The model under review builds one solid part; all positions refer to its coordinate system, in mm. A direction names the side the tool comes from. Round coordinates to 2 decimals unless told otherwise and drop trailing zeros. Write each loop counter-clockwise with the first axis right and the second up, starting at its lowest first coordinate (ties: lowest second). Pieces come first, ordered by that corner, then holes. Notation, with made-up numbers: (-23.5, 8.25) - (24.5, 8.25) arc R14 cw to (24.5, 35.25) - close; hole circle Ø11 at (85, 87.25). An arc over 180 degrees is marked (long way). Write each question's results on one line, items separated by ' | '.
```python
from build123d import *

# Parameters (mm, degrees)
F0_W          = 75
F0_H          = 35
F1_DEPTH      = 3
F4_W          = 10.7173770666
F4_H          = 34.9826700985
F5_DEPTH      = 25
F7_W          = 6
F7_H          = 35
F7_W_2        = 2
F7_H_2        = 28
F8_DEPTH      = 10
F9_DEPTH      = 10
F9_FACE_W     = 6
F9_FACE_H     = 35
F11_W         = 2
F11_H         = 28
F14_DEPTH     = 6
F16_DEPTH     = 25
F17_R         = 2
F18_R         = 0.5
F20_T1_DEPTH  = 12
F20_T4_ANGLE  = 90
F20_T6_ANGLE  = 90
F20_T8_ANGLE  = 90
F20_T10_ANGLE = 90
F21_R         = 1


# Not quite as in the source:
# - a fillet or chamfer that OpenCascade refuses, or shapes differently, is made with other operations: its cross-section is extruded or revolved along the edge and cut away or added
# - a feature of the source that left no trace in its solid (it failed there, or was rolled back) is left out
# - a feature names something its author has since deleted; it is built from what else it names


with BuildPart() as f1:
    # F0 (on Right) → F1 (new body, symmetric)
    with BuildSketch(Plane.YZ):
        with Locations((37.5, 0)):
            Rectangle(F0_W, F0_H)
    extrude(amount=F1_DEPTH, both=True)

    # F4 (on offset) → F5 (cut)
    with BuildSketch(Plane.XZ.offset(-10)):
        Rectangle(F4_W, F4_H)
    extrude(amount=F5_DEPTH, mode=Mode.SUBTRACT)

    # F7 (on face) → F8 (cut)
    with BuildSketch(Plane(origin=(0, 75, 0), x_dir=(-1, 0, 0), z_dir=(0, 1, 0))):
        Rectangle(F7_W, F7_H)
        Rectangle(F7_W_2, F7_H_2, mode=Mode.SUBTRACT)
    extrude(amount=F8_DEPTH, mode=Mode.SUBTRACT)

    # F9 (cut): a face of the model
    f9_faces = [f1.faces().sort_by_distance(p)[0] for p in [
        (0, 75, 0),
    ]]
    extrude(f9_faces, amount=-F9_DEPTH, mode=Mode.SUBTRACT)

    # F9_face (on face) → F12 section 0
    with BuildSketch(Plane(origin=(0, 65, 0), x_dir=(-1, 0, 0), z_dir=(0, 1, 0))):
        Rectangle(F9_FACE_W, F9_FACE_H)
    # F11 (on offset) → F12 section 1
    with BuildSketch(Plane(origin=(0, 75, 0), x_dir=(-1, 0, 0), z_dir=(0, 1, 0))):
        Rectangle(F11_W, F11_H)
    loft()

    # F13 (on Right) → F14 (join, symmetric)
    with BuildSketch(Plane.YZ):
        Polygon((25, 21.5), (0, 21.5), (-25, 21.5), (-25, 0), (-25, -21.5), (0, -21.5), (25, -21.5), (25, 0), align=None)
    extrude(amount=F14_DEPTH, both=True)

    # F15 (on face) → F16 (cut)
    with BuildSketch(Plane(origin=(-6, 0, 0), x_dir=(0, -1, 0), z_dir=(-1, 0, 0))):
        with BuildLine():
            Line((-5, -12.5), (5, -12.5))
            ThreePointArc((5, -12.5), (6.4142135624, -11.9142135624), (7, -10.5))
            Line((7, -10.5), (7, -9.5))
            ThreePointArc((7, -9.5), (6.4142135624, -8.0857864376), (5, -7.5))
            Line((5, -7.5), (-5, -7.5))
            ThreePointArc((-5, -7.5), (-6.4142135624, -8.0857864376), (-7, -9.5))
            Line((-7, -9.5), (-7, -10.5))
            ThreePointArc((-7, -10.5), (-6.4142135624, -11.9142135624), (-5, -12.5))
        make_face()
    extrude(amount=-F16_DEPTH, mode=Mode.SUBTRACT)

    # F17
    f17_edges = [f1.edges().sort_by_distance(p)[0] for p in [
        (6, 0, -7.5),
        (6, -6.414214, -8.085786),
        (6, -7, -10),
        (6, -6.414214, -11.914214),
        (6, 0, -12.5),
        (6, 6.414214, -8.085786),
        (6, 7, -10),
        (6, 6.414214, -11.914214),
        (-6, 0, -7.5),
        (-6, -6.414214, -8.085786),
        (-6, -7, -10),
        (-6, -6.414214, -11.914214),
        (-6, 0, -12.5),
        (-6, 6.414214, -11.914214),
        (-6, 7, -10),
        (-6, 6.414214, -8.085786),
    ]]
    fillet(f17_edges, radius=F17_R)

    # F18
    f18_edges = [f1.edges().sort_by_distance(p)[0] for p in [
        (-6, 0, 21.5),
        (0, -25, 21.5),
        (6, 0, 21.5),
        (0, 25, 21.5),
        (6, 0, -5.5),
        (6, 7.828427, -6.671573),
        (6, -7.828427, -6.671573),
        (6, 9, -10),
        (6, -9, -10),
        (6, 7.828427, -13.328427),
        (6, -7.828427, -13.328427),
        (6, 0, -14.5),
        (6, -25, 0),
        (6, 25, 0),
        (6, 0, -21.5),
        (-6, 0, -5.5),
        (-6, -7.828427, -6.671573),
        (-6, 7.828427, -6.671573),
        (-6, -9, -10),
        (-6, 9, -10),
        (-6, -7.828427, -13.328427),
        (-6, 7.828427, -13.328427),
        (-6, 0, -14.5),
        (-6, 25, 0),
        (-6, -25, 0),
        (-6, 0, -21.5),
    ]]
    fillet(f18_edges, radius=F18_R)

    # F19: F1 across plane


with BuildPart() as f1_1:
    add(f1.part)
    add(f1.part.mirror(Plane.XZ))

    # F20: fillet of radius 1 on 2 edges, made by hand

    # F20_s2 → F20_t1 (cut)
    with BuildSketch(Plane.YZ.offset(-6)):
        with BuildLine():
            ThreePointArc((25, -20.5), (24.7071067812, -21.2071067812), (24, -21.5))
            Line((24, -21.5), (25, -21.5))
            Line((25, -21.5), (25, -20.5))
        make_face()
        with BuildLine():
            ThreePointArc((-25, -20.5), (-24.7071067812, -21.2071067812), (-24, -21.5))
            Line((-24, -21.5), (-25, -21.5))
            Line((-25, -21.5), (-25, -20.5))
        make_face()
    extrude(amount=F20_T1_DEPTH, mode=Mode.SUBTRACT)

    # F20_s3 → F20_t4 (revolve, cut)
    with BuildSketch(Plane.XZ.offset(24)):
        with BuildLine():
            ThreePointArc((-6, -21), (-5.8535533906, -21.3535533906), (-5.5, -21.5))
            Line((-5.5, -21.5), (-6, -21.5))
            Line((-6, -21.5), (-6, -21))
        make_face()
    revolve(axis=Axis((-6, -24, -20.5), (-1, 0, 0)), revolution_arc=F20_T4_ANGLE, mode=Mode.SUBTRACT)

    # F20_s5 → F20_t6 (revolve, cut)
    with BuildSketch(Plane.XY.offset(-20.5)):
        with BuildLine():
            ThreePointArc((6, -24.5), (5.8535533906, -24.8535533906), (5.5, -25))
            Line((5.5, -25), (6, -25))
            Line((6, -25), (6, -24.5))
        make_face()
    revolve(axis=Axis((6, -24, -20.5), (1, 0, 0)), revolution_arc=F20_T6_ANGLE, mode=Mode.SUBTRACT)

    # F20_s7 → F20_t8 (revolve, cut)
    with BuildSketch(Plane.XZ.offset(-24)):
        with BuildLine():
            ThreePointArc((6, -21), (5.8535533906, -21.3535533906), (5.5, -21.5))
            Line((5.5, -21.5), (6, -21.5))
            Line((6, -21.5), (6, -21))
        make_face()
    revolve(axis=Axis((6, 24, -20.5), (1, 0, 0)), revolution_arc=F20_T8_ANGLE, mode=Mode.SUBTRACT)

    # F20_s9 → F20_t10 (revolve, cut)
    with BuildSketch(Plane.XY.offset(-20.5)):
        with BuildLine():
            ThreePointArc((-6, 24.5), (-5.8535533906, 24.8535533906), (-5.5, 25))
            Line((-5.5, 25), (-6, 25))
            Line((-6, 25), (-6, 24.5))
        make_face()
    revolve(axis=Axis((-6, 24, -20.5), (-1, 0, 0)), revolution_arc=F20_T10_ANGLE, mode=Mode.SUBTRACT)

    # F21
    f21_edges = [f1_1.edges().sort_by_distance(p)[0] for p in [
        (3, 45, -17.5),
        (3, 45, 17.5),
        (-3, 45, 17.5),
        (-3, 45, -17.5),
        (-3, -45, 17.5),
        (-3, -45, -17.5),
        (3, -45, -17.5),
        (3, -45, 17.5),
    ]]
    fillet(f21_edges, radius=F21_R)


solid = f1_1.part
```
Q1. Tool access review of faces 4 (the flat face through (0, 0, -12.5)), 5 (the flat face through (0, -45, -17.5)), 6 (the flat face through (0, -45, 17.5)), 7 (the flat face through (-3, -45, 0)): name each direction out of +Z, -Z, +X, -X, +Y, -Y from which nothing blocks a thin tool from reaching the whole face with its end or side.
Evaluation:
face 4: +X, -X | face 5: -Z, +X, -X, -Y | face 6: +Z, +X, -X, -Y | face 7: +Z, -Z, -X, -Y
Q2. We need section A-A (y = 62). State the section outline as (x, z) points.
Evaluation:
outline: (-3, -16.5) arc R1 ccw to (-2, -17.5) - (2, -17.5) arc R1 ccw to (3, -16.5) - (3, 16.5) arc R1 ccw to (2, 17.5) - (-2, 17.5) arc R1 ccw to (-3, 16.5) - close
Q3. Insertion check: P1, Ø6, axis at x = 2, z = 11, coming from the +Y side; P2, Ø1.2, axis at x = -0.5, y = -40, coming from the +Z side; P3, Ø1.2, axis at x = 0, y = 38.5, coming from the -Z side; P4, Ø16.5, axis at y = 37.5, z = -5, coming from the -X side. Each pin has a flat end and moves straight along its axis. Give the tip position at first contact, or say it passes through.
Evaluation:
P1: stops at y = 75 | P2: stops at z = 17.5 | P3: stops at z = -17.5 | P4: stops at x = -3
Q4. For probe 1 along X at (y, z) = (-34, -0.5); probe 2 along Y at (x, z) = (-3.75, 19.5); probe 3 along Z at (x, y) = (-2, 27), list the stretches that pass through material, from the lowest coordinate up.
Evaluation:
probe 1: x = -3 to 3 | probe 2: y = -25 to 25 | probe 3: z = -17.5 to 17.5
Q5. The part is to be moulded in two halves that separate along Z. For faces 1 (the flat face through (0, 45, -17.5)), 2 (the flat face through (0, 0, -7.5)), 3 (the flat face through (6, 0, 0)), say which applies: released by +Z, released by -Z, zero draft, split by the parting line, or undercut.
Evaluation:
face 1: released by -Z | face 2: undercut | face 3: zero draft
